Can you work these out from the model? Positions are in its coordinate system, mm. Round coordinates to 2 decimals unless told otherwise and drop trailing zeros. Write each loop counter-clockwise with the first axis right and the second up, starting at its lowest first coordinate (ties: lowest second). Pieces come first, ordered by that corner, then holes. Notation, with made-up numbers: M -27,-33.5 L -13,-33.5 A17 ccw -13,-15.5 Z; hole C 46,-35.75 d9. An arc over 180 degrees is marked long. Answer in a Markdown table with one row per item. Add a question column.
(1) If I drill on probe 1 along Y at (x, z) = (0, 0.85); probe 2 along Y at (x, z) = (-75, 0.5); probe 3 along Y at (x, z) = (210.5, 0.4), over which ranges is the centre line in solid material (lowest first)?
(2) Suppose I cut it at A-A, the plane z = 0.4. Count the separate pieces of the cut face and the enclosed holes in it, then the cut area to 3 significant figures.
(3) I'm going to push a flat-ended pin straight in: pin 1 (1 mm diameter, centred on x = 203, z = 1, fed in from -Y). Where does the tip first touch, or does it pass through?
(4) If we mould it in two halves opening along X, with no side actions, what happens to faces 1 (the face through (3, 5, 2)), 2 (the face through (224.226, 35.538, 1.014)), 3 (the face through (-146.52, -18.9, 0.99)), 4 (the face through (-211.52, 21.1, 0.99))? For each: released by +X, released by -X, zero draft, split by the parting line, or undercut.
(5) Suppose I cut it at B-B, the plane y = -5.5. Write out the boundary of the cut face in (x, z).
from build123d import *

# Parameters (mm, degrees)
ESQUISSE1_R             = 3.65
BOSS_EXTRU_1_DEPTH      = 2
CONG_1_R                = 18
CONG_2_R                = 20
D_GAGEMENT_M31_D        = 3.4
ENL_V_MAT_EXTRU_1_DEPTH = 234.819122898
D_GAGEMENT_M51_D        = 5.5
D_GAGEMENT_M52_D        = 5.5


with BuildPart() as part:
    # Esquisse1 → Boss.-Extru.1 (new body)
    with BuildSketch(Plane.XY):
        Polygon((-284.958991582, 40), (-150, 40), (150, 40), (284.958991582, 40), (152.479495791, -30), (-152.479495791, -30), align=None)
        with Locations((-215, 20)):
            Circle(ESQUISSE1_R, mode=Mode.SUBTRACT)
        with Locations((-150, -20)):
            Circle(ESQUISSE1_R, mode=Mode.SUBTRACT)
        with Locations((150, -20)):
            Circle(ESQUISSE1_R, mode=Mode.SUBTRACT)
        with Locations((215, 20)):
            Circle(ESQUISSE1_R, mode=Mode.SUBTRACT)
        with Locations((0, -20)):
            Circle(ESQUISSE1_R, mode=Mode.SUBTRACT)
        with Locations((-71.666666667, 20)):
            Circle(ESQUISSE1_R, mode=Mode.SUBTRACT)
        with Locations((71.666666667, 20)):
            Circle(ESQUISSE1_R, mode=Mode.SUBTRACT)
    extrude(amount=BOSS_EXTRU_1_DEPTH)

    # Congé1
    cong_1_edges = [part.edges().sort_by_distance(p)[0] for p in [
        (-284.958991582, 40, 1),
        (284.958991582, 40, 1),
    ]]
    fillet(cong_1_edges, radius=CONG_1_R)

    # Congé2
    cong_2_edges = [part.edges().sort_by_distance(p)[0] for p in [
        (152.479495791, -30, 1),
        (-152.479495791, -30, 1),
    ]]
    fillet(cong_2_edges, radius=CONG_2_R)

    # Dégagement M31 (through all)
    with Locations(Plane(origin=(0, 0, 0), x_dir=(-1, 0, 0), z_dir=(0, 0, -1))):
        with Locations((-200, 33.228756555), (-200, 6.771243445)):
            Hole(D_GAGEMENT_M31_D / 2)

    # Esquisse4 → Enlèv. mat.-Extru.1 (cut, through all)
    with BuildSketch(Plane(origin=(0, 0, 0), x_dir=(-1, 0, 0), z_dir=(0, 0, -1))):
        with BuildLine():
            Line((-229.334149786, 16), (-205, 16))
            ThreePointArc((-205, 16), (-201, 20), (-205, 24))
            Line((-205, 24), (-230.252130857, 24))
            ThreePointArc((-230.252130857, 24), (-230.246241418, 19.948007721), (-229.334149786, 16))
        make_face()
        with BuildLine():
            Line((-210, 31.528756555), (-190, 31.528756555))
            ThreePointArc((-190, 31.528756555), (-188.3, 33.228756555), (-190, 34.928756555))
            Line((-190, 34.928756555), (-210, 34.928756555))
            ThreePointArc((-210, 34.928756555), (-211.7, 33.228756555), (-210, 31.528756555))
        make_face()
        with BuildLine():
            Line((-210, 5.071243445), (-190, 5.071243445))
            ThreePointArc((-190, 5.071243445), (-188.3, 6.771243445), (-190, 8.471243445))
            Line((-190, 8.471243445), (-210, 8.471243445))
            ThreePointArc((-210, 8.471243445), (-211.7, 6.771243445), (-210, 5.071243445))
        make_face()
    extrude(amount=-ENL_V_MAT_EXTRU_1_DEPTH, mode=Mode.SUBTRACT)

    # Dégagement M51 (through all)
    with Locations(Plane(origin=(0, 0, 0), x_dir=(-1, 0, 0), z_dir=(0, 0, -1))):
        with Locations((143.333333333, 20), (0, 20), (-143.333333333, 20)):
            Hole(D_GAGEMENT_M51_D / 2)

    # Dégagement M52 (through all)
    with Locations(Plane.XY.offset(2)):
        with Locations((-75, -20), (75, -20)):
            Hole(D_GAGEMENT_M52_D / 2)


solid = part.part
Calculated:
| question | item | result |
|---|---|---|
| 1 | probe 1 | -30 to -23.65, -16.35 to 17.25, 22.75 to 40 |
| 1 | probe 2 | -30 to -22.75, -17.25 to 18.51, 21.49 to 40 |
| 1 | probe 3 | 0.66 to 5.15, 8.4 to 16, 24 to 31.6, 34.85 to 40 |
| 2 | separate pieces | 1 |
| 2 | enclosed holes | 13 |
| 2 | area | 28,100 mm² |
| 3 | pin 1 | y = -3.57 |
| 4 | face 1 | zero draft |
| 4 | face 2 | released by +X |
| 4 | face 3 | undercut |
| 4 | face 4 | undercut |
| 5 | outline | M -198.85,0 L 198.85,0 L 198.85,2 L -198.85,2 Z |
